Source: CAD feature listing. Evaluate the final solid. Frame: model axes, mm. Face numbers are marked on the shaded views. A direction names the side the tool comes from. Give positions to 0.01 mm unless a question says otherwise; leave off trailing zeros. Write each loop counter-clockwise with the first axis right and the second up, starting at its lowest first coordinate (ties: lowest second). Pieces come first, ordered by that corner, then holes. Notation, with made-up numbers: (16.5, 25.5) -> (44.5, 25.5) arc R17 cw to (44.5, 34.5) -> close; hole circle Ø8 at (15, 44). An arc over 180 degrees is marked (long way). Use a Markdown table: item, result. Add a question column.
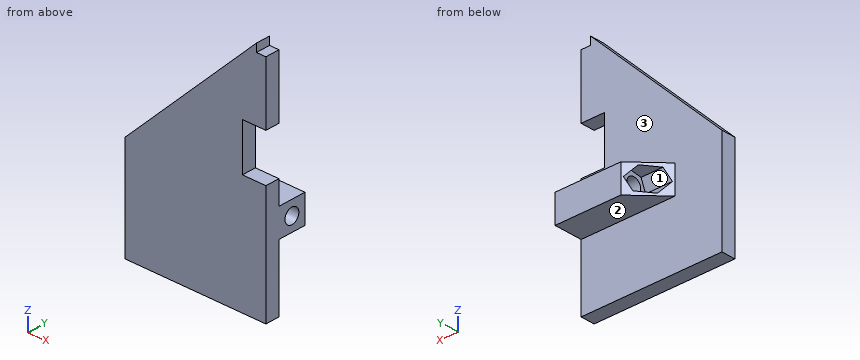
Autodesk Inventor part; units mm, degrees
ref_plane "YZ Plane" through (0, 0, 0) normal (1, 0, 0) x (0, 1, 0)
ref_plane "XZ Plane" through (0, 0, 0) normal (0, 1, 0) x (-1, 0, 0)
ref_plane "XY Plane" through (0, 0, 0) normal (0, 0, 1) x (1, 0, 0)
sketch "Szkic1" plane through (0, 0, 0) normal (0, 1, 0) x (-1, 0, 0)
  line L0 (0, 8) -> (0, 56.3)
  line L1 (0, 58) -> (2, 58) construction
  line L2 (2, 58) -> (2, 56.3) construction
  line L3 (2, 56.3) -> (0, 56.3) construction
  line L4 (0, 56.3) -> (0, 58) construction
  line L5 (30, 8) -> (30, 66.5) construction
  line L6 (2, 58) -> (30, 30)
  line L7 (2, 58) -> (41.598, 58) construction
  line L8 (30, 30) -> (30, 8)
  line L9 (2, 58) -> (2, 56.3)
  line L10 (0, 56.3) -> (2, 56.3)
  line L11 (2, 56.3) -> (2, 54.3) construction
  line L12 (0, 43) -> (5, 43)
  line L13 (5, 43) -> (5, 33)
  line L14 (5, 33) -> (0, 33)
  line L15 (0, 33) -> (0, 43)
  line L16 (30, 8) -> (0, 8)
  line L17 (30, 8) -> (30, 30)
  point P0 (0, 0)
  point P1 (0, 33)
  dimension "d0" = 58
  dimension "d1" = 2
  dimension "d2" = 1.7
  dimension "d4" = 45
  dimension "d7" = 2
  dimension "d8" = 5
  dimension "d9" = 10
  dimension "d13" = 30
  dimension "d14" = 22
  dimension "d15" = 58.5
  dimension "d16" = 30
  dimension "d17" = 25
  dimension "d18" = 8
extrude "Wyciągnięcie proste1" add sketch "Szkic1" along normal blind 3
extrude "Wyciągnięcie proste2" cut sketch "Szkic1" along normal blind 10 contours L0 L12 L13 L14
sketch "Sketch2" plane through (0, 0, 8) normal (1, 0, 0) x (0, 0, -1)
  line L0 (-25, 3) -> (0, 3)
  line L1 (-20, 3) -> (-14, 3)
  line L2 (-14, 3) -> (-14, 9)
  line L3 (-14, 9) -> (-20, 9)
  line L4 (-20, 9) -> (-20, 3)
  line L5 (-14.4598, 4.9465) -> (-16.6422, 3.2734)
  line L6 (-16.6422, 3.2734) -> (-19.1824, 4.3268)
  line L7 (-19.1824, 4.3268) -> (-19.5402, 7.0535)
  line L8 (-19.5402, 7.0535) -> (-17.3578, 8.7266)
  line L9 (-17.3578, 8.7266) -> (-14.8176, 7.6732)
  line L10 (-14.8176, 7.6732) -> (-14.4598, 4.9465)
  point P0 (8, 0)
  point P1 (-17, 6)
  point P2 (-17, 6)
  dimension "d19" = 6
  dimension "d20" = 6
  dimension "d21" = 5
  dimension "d24" = 3
  dimension "d25" = 3
  dimension "d29" = 1.6731
  dimension "d30" = 2.75
extrude "Extrusion3" add sketch "Sketch2" against normal blind 20 contours L4 L3 L2 L0 | L5 L6 L7 L8 L9 L10
extrude "Extrusion4" cut sketch "Sketch2" along normal blind 6 from surface at -20 contours L5 L6 L7 L8 L9 L10
chamfer "Chamfer2" distance 6 angle 45 1 edges at (-20, 9, 25)
hole "Hole1" at (0, 6, 25) direction (-1, 0, 0) diameter 3.2 depth 30
properties part number "ScianaBocznaPEMv2"
(1) Cut plane B-B on x = -8. Return the cut outline in (y, z), then the cut area to 3 significant figures.
(2) Cut plane C-C on y = 6. Return the cut outline in (x, z).
(3) Material intervals for L1, parallel to Z at x = -10.75, y = 6; L2, parallel to Y at x = -8.5, z = 25; L3, parallel to Z at x = -12, y = 3.25, sorted ascending.
(4) Cut plane D-D on z = 33.5. Return the cut outline in (x, y), then the cut area to 3 significant figures.
(5) Access query for the marked faces 1, 2 and 3. Directions: +Z, -Z, +X, -X, +Y, -Y. A direction counts if a zero-diameter tool reaches every point of the face in a straight line with its end or side. Return the directions, or none.
(6) First-contact query: pin 1 Ø3 at (x, y) = (-7, 5.5) entering from +Z; pin 2 Ø3 at (y, z) = (6, 25) entering from +X; pin 3 Ø0.6 at (x, y) = (-1, 2) entering from +Z; pin 4 Ø1.5 at (y, z) = (2, 40) entering from +X. Flat tips, straight axial feed; report the tip coordinate or a pass-through.
(7) Cut plane A-A on y = 1. Return the cut outline in (x, z), then the cut area to 3 significant figures.
Output:
| question | item | result |
|---|---|---|
| 1 | outline | (0, 8) -> (3, 8) -> (3, 22) -> (9, 22) -> (9, 28) -> (3, 28) -> (3, 52) -> (0, 52) -> close; hole circle Ø3.2 at (6, 25) |
| 1 | area | 160 mm^2 |
| 2 | outline | (-17, 22) -> (0, 22) -> (0, 23.4) -> (-14, 23.4) -> (-14, 22.6) -> (-17, 22.6) -> close; (-17, 27.4) -> (-14, 27.4) -> (-14, 26.6) -> (0, 26.6) -> (0, 28) -> (-17, 28) -> close |
| 3 | L1 | 22 to 23.4, 26.6 to 28 |
| 3 | L2 | 0 to 4.4, 7.6 to 9 |
| 3 | L3 | 22 to 28 |
| 4 | outline | (-26.5, 0) -> (-5, 0) -> (-5, 3) -> (-26.5, 3) -> close |
| 4 | area | 64.5 mm^2 |
| 5 | face 1 | -X |
| 5 | face 2 | -Z, +X, -X, +Y |
| 5 | face 3 | -X, +Y |
| 6 | pin 1 | z = 28 |
| 6 | pin 2 | through |
| 6 | pin 3 | z = 56.3 |
| 6 | pin 4 | x = -5 |
| 7 | outline | (-30, 8) -> (0, 8) -> (0, 33) -> (-5, 33) -> (-5, 43) -> (0, 43) -> (0, 56.3) -> (-2, 56.3) -> (-2, 58) -> (-30, 30) -> close |
| 7 | area | 1,050 mm^2 |
